Autodesk Inventor part; units mm, degrees
ref_plane "YZ Plane" through (0, 0, 0) normal (1, 0, 0) x (0, 1, 0)
ref_plane "XZ Plane" through (0, 0, 0) normal (0, 1, 0) x (-1, 0, 0)
ref_plane "XY Plane" through (0, 0, 0) normal (0, 0, 1) x (1, 0, 0)
sketch "Sketch1" plane through (0, 0, 0) normal (0, 0, 1) x (1, 0, 0)
  circle A0 centre (-790.1228, -10.9134) radius 9.525
  ellipse E0 centre (61.5218, 18.65) end of major axis (52.5416, 18.65) minor radius 6.35 (61.5218, 25) -> (52.5416, 18.65) ccw
  line L0 (61.5218, 25) -> (114.272, 25)
  ellipse E1 centre (114.272, 18.65) end of major axis (105.2917, 18.65) minor radius 6.35 (123.2522, 18.65) -> (114.272, 25) ccw
  line L1 (123.2522, 18.65) -> (123.2522, -18.65)
  ellipse E2 centre (114.272, -18.65) end of major axis (105.2917, -18.65) minor radius 6.35 (114.272, -25) -> (123.2522, -18.65) ccw
  line L2 (114.272, -25) -> (61.5218, -25)
  ellipse E3 centre (61.5218, -18.65) end of major axis (52.5416, -18.65) minor radius 6.35 (52.5416, -18.65) -> (61.5218, -25) ccw
  line L3 (52.5416, -18.65) -> (52.5416, 18.65)
  line L4 (114.272, 21.825) -> (61.5218, 21.825)
  ellipse E4 centre (61.5218, 18.65) end of major axis (57.0317, 18.65) minor radius 3.175 (61.5218, 21.825) -> (57.0317, 18.65) ccw
  line L5 (57.0317, 18.65) -> (57.0317, -18.65)
  ellipse E5 centre (61.5218, -18.65) end of major axis (57.0317, -18.65) minor radius 3.175 (57.0317, -18.65) -> (61.5218, -21.825) ccw
  line L6 (61.5218, -21.825) -> (114.272, -21.825)
  ellipse E6 centre (114.272, -18.65) end of major axis (109.7818, -18.65) minor radius 3.175 (114.272, -21.825) -> (118.7621, -18.65) ccw
  line L7 (118.7621, -18.65) -> (118.7621, 18.65)
  ellipse E7 centre (114.272, 18.65) end of major axis (109.7818, 18.65) minor radius 3.175 (118.7621, 18.65) -> (114.272, 21.825) ccw
  circle A1 centre (17.6912, 0) radius 5
  circle A2 centre (17.6912, 0) radius 10
  line L8 (15.357, 9.7238) -> (52.5416, 18.65)
  line L9 (52.5416, -18.65) -> (15.357, -9.7238)
  dimension "d4" = 20
extrude "Extrusion1" add sketch "Sketch1" along normal blind 6 contours L3 L9 A2 L8 | A2
chamfer "Chamfer1" distance 5 angle 45 1 edges at (52.5416, 0, 6)
thicken "Thicken1" operation add thickness 3 both sides no extend neighbours yes toward (-0.7071068, 0, -0.7071068) faces at (50.8749, 5.8166, 2.6667)
sketch "Sketch2" plane through (0, 0, 0) normal (0, 0, -1) x (-1, 0, 0)
  line L0 (-49.2989, -17.8716) -> (-49.2989, 17.8716)
  line L1 (-15.357, -9.7238) -> (-49.2989, -17.8716)
  arc A0 (-15.357, -9.7238) -> (-15.357, 9.7238) centre (-17.6912, 0) ccw
  line L2 (-49.2989, 17.8716) -> (-15.357, 9.7238)
  circle A1 centre (-17.6912, 0) radius 5
  line L3 (-112.6912, -35.5) -> (-42.6912, -35.5)
  line L4 (-42.6912, -35.5) -> (-42.6912, 35.5)
  line L5 (-42.6912, 35.5) -> (-112.6912, 35.5)
  line L6 (-112.6912, -35.5) -> (-42.6912, 35.5) construction
  line L7 (-42.6912, -35.5) -> (-112.6912, 35.5) construction
  line L8 (-42.6912, 35.5) -> (-11.061, 7.486)
  arc A2 (-15.357, -9.7238) -> (-15.357, 9.7238) centre (-17.6912, 0) ccw
  line L9 (-42.6912, -35.5) -> (-11.061, -7.486)
  line L10 (-102.6912, -25.5) -> (-52.6912, -25.5)
  line L11 (-52.6912, -25.5) -> (-52.6912, 25.5)
  line L12 (-52.6912, 25.5) -> (-102.6912, 25.5)
  line L13 (-102.6912, -25.5) -> (-52.6912, 25.5) construction
  line L14 (-52.6912, -25.5) -> (-102.6912, 25.5) construction
  line L15 (-102.6912, 25.5) -> (-112.6912, 25.5)
  line L16 (-112.6912, -25.5) -> (-102.6912, -25.5)
  line L17 (-112.6912, 35.5) -> (-112.6912, 25.5)
  line L18 (-112.6912, -25.5) -> (-112.6912, -35.5)
  line L19 (-49.2989, -17.8716) -> (-49.2989, 17.8716)
  point P0 (0, 0)
  point P1 (-77.6912, 0)
  point P2 (-49.2989, 0)
  point P3 (-77.6912, 0)
  point P4 (-11.061, -7.486)
  point P5 (-11.061, 7.486)
  point P6 (-49.2989, 0)
  point P7 (-52.6912, 0)
  dimension "d13" = 51
  dimension "d14" = 35
  dimension "d15" = 10
  dimension "d16" = 50
  dimension "d17" = 10
  dimension "d30" = 71
extrude "Extrusion2" add sketch "Sketch2" against normal up to surface (6 mm away)
chamfer "Chamfer2" distance 5 angle 45 2 edges at (112.6912, 35.5, 3) (112.6912, -35.5, 3)
sketch "Sketch3" plane through (0, 0, 0) normal (0, 0, -1) x (-1, 0, 0)
  line L0 (-107.6912, -35.5) -> (-112.6912, -30.5)
  line L1 (-107.6912, -35.5) -> (-42.6912, -35.5)
  line L2 (-42.6912, -35.5) -> (-11.061, -7.486)
  arc A0 (-11.061, -7.486) -> (-11.061, 7.486) centre (-17.6912, 0) ccw
  line L3 (-11.061, 7.486) -> (-42.6912, 35.5)
  line L4 (-42.6912, 35.5) -> (-107.6912, 35.5)
  line L5 (-112.6912, 30.5) -> (-107.6912, 35.5)
  line L6 (-112.6912, 30.5) -> (-112.6912, 25.5)
  line L7 (-112.6912, 25.5) -> (-52.6912, 25.5)
  line L8 (-52.6912, 25.5) -> (-52.6912, -25.5)
  line L9 (-52.6912, -25.5) -> (-112.6912, -25.5)
  line L10 (-112.6912, -25.5) -> (-112.6912, -30.5)
  circle A1 centre (-17.6912, 0) radius 5
  line L11 (-52.6912, 25.5) -> (-52.6912, -25.5)
  circle A2 centre (-52.6912, 25.5) radius 1.5
  circle A3 centre (-52.6912, -25.5) radius 1.5
  point P0 (0, 0)
  dimension "d23" = 3
  dimension "d24" = 3
extrude "Extrusion3" cut sketch "Sketch3" against normal through all contours A3 L8 L9 | L9 L8 A3 | A2 L7 L8 | L8 L7 A2
fillet "Fillet1" radius 2 4 edges at (52.6912, -24, 3) (54.1912, -25.5, 3) (54.1912, 25.5, 3) (52.6912, 24, 3)
fillet "Fillet2" radius 2 6 edges at (107.6912, -35.5, 3) (112.6912, -30.5, 3) (107.6912, 35.5, 3) (112.6912, 30.5, 3) (112.6912, 25.5, 3) (112.6912, -25.5, 3)
fillet "Fillet3" radius 20 2 edges at (42.6912, 35.5, 3) (42.6912, -35.5, 3)
properties part number "FRC003-1"
Source: CAD feature listing. Evaluate the final solid. Frame: model axes, mm. A direction names the side the tool comes from. Give positions to 0.01 mm unless a question says otherwise; leave off trailing zeros. Write each loop counter-clockwise with the first axis right and the second up, starting at its lowest first coordinate (ties: lowest second). Pieces come first, ordered by that corner, then holes.
1. Access query for faces 1 (the face through (83, 25.5, 3)), 2 (the face through (51.6, 26.53, 2.96)). Directions: +Z, -Z, +X, -X, +Y, -Y. A direction counts if a zero-diameter tool reaches every point of the face in a straight line with its end or side. Return the directions, or none.
2. Pull-direction query (X, two-part tool) for faces 3 (the face through (48, 0, 0)), 4 (the face through (112.09, 26.07, 3.04)), 5 (the face through (12.696, -0.22, 2.958)), 6 (the face through (51.66, -26.59, 2.96)); classes: +X half, -X half, draft (parallel to the pull), parting line (faces both ways), or undercut.
3. First-contact query: pin 1 (3 mm diameter, centred on y = -2, z = 3, fed in from +X). Flat tip, straight axial feed; report the tip coordinate or a pass-through.
4. Section query C-C (z = 3.85). Return the cut outline in (x, y), then the cut area to 3 significant figures.
5. Material intervals for line 1 along Y through (x, z) = (89.5, 2.45); line 2 along X through (y, z) = (0, 2.65); line 3 along Y through (x, z) = (37, 5.15), sorted ascending.
6. Section query A-A (y = 0). Return the cut outline in (x, z), then the cut area to 3 significant figures.
7. Section query B-B (x = 89). Return the cut outline in (y, z), then the cut area to 3 significant figures.
8. Section query D-D (x = 44.5). Return the cut outline in (y, z).
Output values:
1. face 1: +Z, -Z, +X
1. face 2: +Z, -Z
2. face 3: draft
2. face 4: +X half
2. face 5: undercut
2. face 6: undercut
3. pin 1: stops at x = 52.69
4. outline: (11.06, -7.49) - (37.01, -30.47) arc R20 ccw to (50.27, -35.5) - (106.86, -35.5) arc R2 ccw to (108.28, -34.91) - (112.11, -31.09) arc R2 ccw to (112.69, -29.67) - (112.69, -27.5) arc R2 ccw to (110.69, -25.5) - (55.56, -25.5) arc R2 ccw to (53.92, -26.36) arc R1.5 cw (long way) to (51.83, -24.27) arc R2 ccw to (52.69, -22.63) - (52.69, 22.63) arc R2 ccw to (51.83, 24.27) arc R1.5 cw (long way) to (53.92, 26.36) arc R2 ccw to (55.56, 25.5) - (110.69, 25.5) arc R2 ccw to (112.69, 27.5) - (112.69, 29.67) arc R2 ccw to (112.11, 31.09) - (108.28, 34.91) arc R2 ccw to (106.86, 35.5) - (50.27, 35.5) arc R20 ccw to (37.01, 30.47) - (11.06, 7.49) arc R10 ccw to start; hole circle Ø10 at (17.69, 0)
4. area: 3,170 mm2
5. line 1: y = -35.5 to -25.5, 25.5 to 35.5
5. line 2: x = 7.69 to 12.69, 22.69 to 52.69
5. line 3: y = -30.46 to 30.46
6. outline: (7.69, 0) - (12.69, 0) - (12.69, 6) - (7.69, 6) - close; (22.69, 0) - (52.69, 0) - (52.69, 6) - (22.69, 6) - close
6. area: 210 mm2
7. outline: (-35.5, 0) - (-25.5, 0) - (-25.5, 6) - (-35.5, 6) - close; (25.5, 0) - (35.5, 0) - (35.5, 6) - (25.5, 6) - close
7. area: 120 mm2
8. outline: (-34.65, 0) - (34.65, 0) - (34.65, 6) - (-34.65, 6) - close
